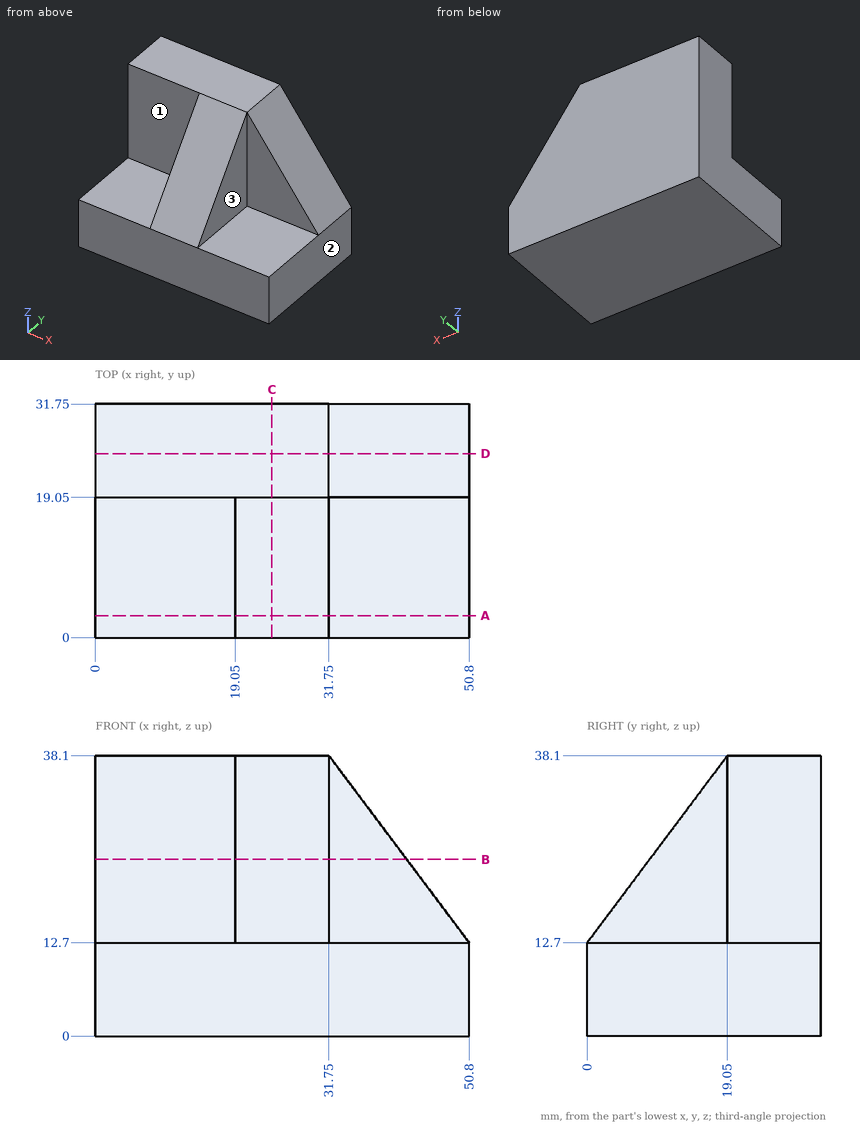
Print and shaded views of the part. All mm, measured from the part's lowest x, y and z. A direction names the side the tool comes from. Give positions to 0.01 mm unless a question says otherwise; leave off trailing zeros. Order: outer loops, then holes, each group sorted by start corner. A loop starts at its lowest first (then second) coordinate and runs counter-clockwise, first axis right, second up. Notation, with made-up numbers: (12, 41.5) - (41, 41.5) arc R21 ccw to (41, 57.5) - close; hole circle Ø8 at (45, -37). An arc over 180 degrees is marked (long way). One line per item, written item: value.
Item 1: Slice it at C-C (x = 24). List the corners of the cut face in (y, z), then the cut area to 3 significant figures.
Response values:
outline: (0, 0) - (31.75, 0) - (31.75, 38.1) - (19.05, 38.1) - (0, 12.7) - close
area: 968 mm2
Item 2: Pin check, flat tips, straight feed: pin 1 Ø9.5 at (y, z) = (10, 21.5) entering from -X; pin 2 Ø5.5 at (x, z) = (13.5, 27.5) entering from -Y; pin 3 Ø10 at (x, y) = (33.5, 13) entering from +Z. Stop position of each tip, or through.
Response values:
pin 1: x = 19.05
pin 2: y = 19.05
pin 3: z = 36.28
Item 3: Tool access for the marked faces 1, 2 and 3: list every direction of +Z, -Z, +X, -X, +Y, -Y with a clear straight run to the whole face (end or side of a thin tool).
Response values:
face 1: +Z, -X, -Y
face 2: +Z, -Z, +X, +Y, -Y
face 3: +Z, +X, -Y
Item 4: Slice it at B-B (z = 24). List the corners of the cut face in (x, y) (3 decimals), then the cut area to 3 significant figures.
Response values:
outline: (0, 19.05) - (19.05, 19.05) - (19.05, 8.475) - (31.75, 8.475) - (31.75, 19.05) - (42.325, 19.05) - (42.325, 31.75) - (0, 31.75) - close
area: 672 mm2
Item 5: Slice it at A-A (y = 3). List the corners of the cut face in (x, z).
Response values:
outline: (0, 0) - (50.8, 0) - (50.8, 12.7) - (31.75, 12.7) - (31.75, 16.7) - (19.05, 16.7) - (19.05, 12.7) - (0, 12.7) - close
Item 6: Slice it at D-D (y = 25). List the corners of the cut face in (x, z), then the cut area to 3 significant figures.
Response values:
outline: (0, 0) - (50.8, 0) - (50.8, 12.7) - (31.75, 38.1) - (0, 38.1) - close
area: 1,690 mm2
Item 7: Wall check: line 1 (Y direction, x = 14.5, z = 16); line 2 (Z direction, x = 34.5, y = 11). Give the ranges that are in metal, low to high.
Response values:
line 1: 19.05 to 31.75
line 2: 0 to 12.7
